CAD build for the part. Positions are in the model's coordinates, mm. A direction names the side the tool comes from. Coordinates: 2 decimals unless noted, no trailing zeros. Loops run counter-clockwise (first coordinate to the right, second up) from the corner with the lowest first, then second, coordinate; pieces in that order, holes last. Notation, with made-up numbers: (53.5, -22.75) -> (62.5, -22.75) arc R17 cw to (62.5, -12.75) -> close; hole circle Ø10 at (21, 48). An arc over 180 degrees is marked (long way). Answer as a JSON object with one key per item and string values. Group by question number.
from build123d import *

# Parameters (mm, degrees)
SKETCH2_R           = 3.429
BOSS_EXTRUDE1_DEPTH = 19.05
BOSS_EXTRUDE2_START = 19.05
SKETCH3_R           = 8.1915
SKETCH3_R_2         = 3.429
SKETCH3_R_3         = 6.35
BOSS_EXTRUDE2_DEPTH = 19.05
BOSS_EXTRUDE5_START = 3.429
SKETCH4_R           = 6.35
SKETCH4_R_2         = 3.429
BOSS_EXTRUDE5_DEPTH = 3.429
BOSS_EXTRUDE6_START = -19.05
BOSS_EXTRUDE6_DEPTH = 6.35


with BuildPart() as part:
    # Sketch2 → Boss-Extrude1 (new body)
    with BuildSketch(Plane(origin=(0, 0, 0), x_dir=(1, 0, 0), z_dir=(0, 1, 0))):
        with BuildLine():
            Line((-84.142567987, -15.875), (-42.857432013, -15.875))
            ThreePointArc((-42.857432013, -15.875), (-40.864863591, -16.578098691), (-39.754797373, -18.375994594))
            ThreePointArc((-39.754797373, -18.375994594), (-31.75, -24.828560646), (-23.745202627, -18.375994594))
            ThreePointArc((-23.745202627, -18.375994594), (-22.635136409, -16.578098691), (-20.642567987, -15.875))
            Line((-20.642567987, -15.875), (-19.05, -15.875))
            ThreePointArc((-19.05, -15.875), (-16.80493597, -16.80493597), (-15.875, -19.05))
            Line((-15.875, -19.05), (-15.875, -70.612060646))
            ThreePointArc((-15.875, -70.612060646), (-14.94506403, -72.857124676), (-12.7, -73.787060646))
            Line((-12.7, -73.787060646), (-6.35, -73.787060646))
            ThreePointArc((-6.35, -73.787060646), (-0.091449146, -68.510858211), (-4.233333333, -61.450223232))
            ThreePointArc((-4.233333333, -61.450223232), (-5.767376644, -60.28989163), (-6.35, -58.456804525))
            Line((-6.35, -58.456804525), (-6.35, -12.7))
            ThreePointArc((-6.35, -12.7), (-8.209871939, -8.209871939), (-12.7, -6.35))
            Line((-12.7, -6.35), (-128.5875, -6.35))
            ThreePointArc((-128.5875, -6.35), (-137.567756121, -10.069743879), (-141.2875, -19.05))
            Line((-141.2875, -19.05), (-141.2875, -61.948583794))
            ThreePointArc((-141.2875, -61.948583794), (-140.35756403, -64.193647824), (-138.1125, -65.123583794))
            Line((-138.1125, -65.123583794), (-134.9375, -65.123583794))
            ThreePointArc((-134.9375, -65.123583794), (-132.69243597, -64.193647824), (-131.7625, -61.948583794))
            Line((-131.7625, -61.948583794), (-131.7625, -22.225))
            ThreePointArc((-131.7625, -22.225), (-129.90262806, -17.734871939), (-125.4125, -15.875))
            Line((-125.4125, -15.875), (-106.357432013, -15.875))
            ThreePointArc((-106.357432013, -15.875), (-104.364863591, -16.578098691), (-103.254797373, -18.375994594))
            ThreePointArc((-103.254797373, -18.375994594), (-95.25, -24.828560646), (-87.245202627, -18.375994594))
            ThreePointArc((-87.245202627, -18.375994594), (-86.135136409, -16.578098691), (-84.142567987, -15.875))
        make_face()
        with Locations(Location((-95.25, -16.637060646, 0), (0, 0, 270))):
            Circle(SKETCH2_R, mode=Mode.SUBTRACT)
        with Locations(Location((-31.75, -16.637060646, 0), (0, 0, 270))):
            Circle(SKETCH2_R, mode=Mode.SUBTRACT)
        with Locations(Location((-6.35, -67.437060646, 0), (0, 0, 270))):
            Circle(SKETCH2_R, mode=Mode.SUBTRACT)
    extrude(amount=-BOSS_EXTRUDE1_DEPTH)

    # Sketch3 → Boss-Extrude2 (add)
    # profile 1 of 3: a face of its own
    with BuildSketch(Plane(origin=(0, 0, 0), x_dir=(1, 0, 0), z_dir=(0, 1, 0)).offset(BOSS_EXTRUDE2_START)):
        with Locations(Location((-95.25, -16.637060646, 0), (0, 0, 270))):
            Circle(SKETCH3_R)
        with Locations(Location((-95.25, -16.637060646, 0), (0, 0, 270))):
            Circle(SKETCH3_R_2, mode=Mode.SUBTRACT)
    # profile 2 of 3: a face of its own
    with BuildSketch(Plane(origin=(0, 0, 0), x_dir=(1, 0, 0), z_dir=(0, 1, 0)).offset(BOSS_EXTRUDE2_START)):
        with Locations(Location((-31.75, -16.637060646, 0), (0, 0, 270))):
            Circle(SKETCH3_R)
        with Locations(Location((-31.75, -16.637060646, 0), (0, 0, 270))):
            Circle(SKETCH3_R_2, mode=Mode.SUBTRACT)
    # profile 3 of 3: a face of its own
    with BuildSketch(Plane(origin=(0, 0, 0), x_dir=(1, 0, 0), z_dir=(0, 1, 0)).offset(BOSS_EXTRUDE2_START)):
        with Locations(Location((-6.35, -67.437060646, 0), (0, 0, 270))):
            Circle(SKETCH3_R_3)
        with Locations(Location((-6.35, -67.437060646, 0), (0, 0, 270))):
            Circle(SKETCH3_R_2, mode=Mode.SUBTRACT)
    extrude(amount=-BOSS_EXTRUDE2_DEPTH)

    # Sketch4 → Boss-Extrude5 (add)
    with BuildSketch(Plane(origin=(0, 19.05, 0), x_dir=(1, 0, 0), z_dir=(0, 1, 0)).offset(BOSS_EXTRUDE5_START)):
        with Locations(Location((-6.35, -67.437060646, 0), (0, 0, 270))):
            Circle(SKETCH4_R)
        with Locations(Location((-6.35, -67.437060646, 0), (0, 0, 270))):
            Circle(SKETCH4_R_2, mode=Mode.SUBTRACT)
    extrude(amount=-BOSS_EXTRUDE5_DEPTH)

    # Sketch6 → Boss-Extrude6 (add)
    with BuildSketch(Plane(origin=(0, 0, 0), x_dir=(1, 0, 0), z_dir=(0, 1, 0)).offset(BOSS_EXTRUDE6_START)):
        Polygon((-112.7125, -15.875), (-131.7625, -47.625), (-131.7625, -15.875), align=None)
    extrude(amount=BOSS_EXTRUDE6_DEPTH)


solid = part.part
Item 1: Band-saw the part on C-C, the plane y = -7. Count the separate pieces of the cut face and the enclosed holes in it, and give its area (3 significant figures).
Item 2: 3-axis set-ups, long thin cutter, end or side, ignore diameter. For faces 1 (the cylindrical face through (-140.38, -9.39, 64.17)), 2 (the cylindrical face through (-40.89, -9.39, 16.56)), 3 (the flat face through (-116, -7, 15.875)): which of +Z, -Z, +X, -X, +Y, -Y reach the whole face in a straight line?
Item 3: Band-saw the part on A-A, the plane y = 6. List the corners of the cut face in (x, z).
Item 4: Pull direction Z, two halves, no side cores. Call faces 4 (the cylindrical face through (-98.6, 0.3, 15.9)), 5 (the cylindrical face through (-129.95, -6.26, 17.78)), 6 (the flat face through (-126, -12.7, 24)), 7 (the cylindrical face through (-0.996, 6.62, 70.851)): +Z half, -Z half, draft (parallel to the pull), parting line (faces both ways), or undercut.
Item 5: Drill centre lines: L1, parallel to X at y = -5.5, z = 65.5 (3 decimals); L2, parallel to X at y = -12, z = 17; L3, parallel to Y at x = -58, z = 13. Where is each one in solid material? Low to high.
Item 6: Band-saw the part on D-D, the plane x = -62. List the corners of the cut face in (y, z) (3 decimals).
Item 7: Flat gauge pins, fed straight in: P1, Ø12, axis at x = -41.5, y = 6, coming from the +Z side; P2, Ø15, axis at x = -57, y = -13.5, coming from the +Z side (3 decimals); P3, Ø10, axis at x = -22, y = 15, coming from the +Z side. Where does each tip first touch, or does it go through?
Reply:
{
 "1": {"separate pieces": "1", "enclosed holes": "3", "area": "2,460 mm²"},
 "2": {"face 1": "+Z, -X, +Y, -Y", "face 2": "+Z, +Y, -Y", "face 3": "+Z, +Y"},
 "3": {"outline": "circle Ø16.38 at (-95.25, 16.64); circle Ø16.38 at (-31.75, 16.64); circle Ø12.7 at (-6.35, 67.44); hole circle Ø6.86 at (-95.25, 16.64); hole circle Ø6.86 at (-31.75, 16.64); hole circle Ø6.86 at (-6.35, 67.44)"},
 "4": {"face 4": "undercut", "face 5": "+Z half", "face 6": "draft", "face 7": "parting line"},
 "5": {"L1": "-15.875 to -9.179, -3.521 to -0.303", "L2": "-141.12 to -129.02, -103.93 to -98.66, -91.84 to -86.57, -40.43 to -35.16, -28.34 to -23.07, -16.63 to -6.35", "L3": "-19.05 to 0"},
 "6": {"outline": "(-19.05, 6.35) -> (0, 6.35) -> (0, 15.875) -> (-19.05, 15.875) -> close"},
 "7": {"P1": "z = 23.92", "P2": "z = 15.875", "P3": "z = 23.31"}
}
